Answer from the drawing. Dimensions are ordinates in mm from the lowest x, y and z of the part. Coordinates: 2 decimals unless noted, no trailing zeros. Write each loop counter-clockwise with the first axis right and the second up, starting at its lowest first coordinate (ties: lowest second). Pieces come first, ordered by that corner, then holes. Notation, with made-up numbers: (9.25, 78.25) - (20.25, 78.25) arc R16 ccw to (20.25, 83.25) - close; hole circle Ø1 at (32, -9.75). An arc over 180 degrees is marked (long way). Use CSV: the item, a comma, the result in double quotes. Start each with the question number.
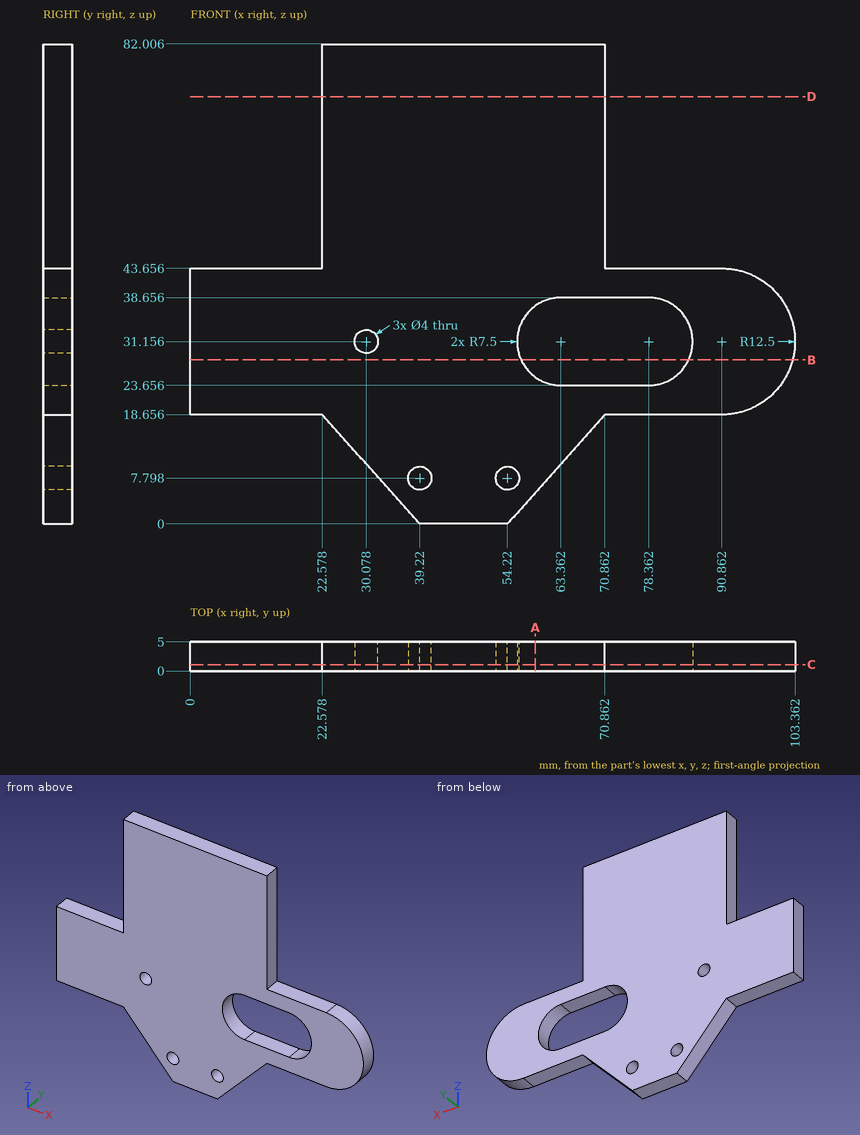
Item 1: A cutting plane is placed at C-C (y = 1.1). Determine the outline of the cut face in (x, z) (1 decimal).
Item 2: A cutting plane is placed at B-B (z = 28). Determine the outline of the cut face in (x, y) (1 decimal).
Item 3: Each of these flat-tipped pins is pushed along its axis until it touches: pin 1 (2.5 mm diameter, centred on x = 78, y = 3, fed in from +Z); pin 2 (1.5 mm diameter, centred on x = 12, y = 3.5, fed in from -Z); pin 3 (2.5 mm diameter, centred on x = 72, y = 1.5, fed in from -Z); pin 4 (2.5 mm diameter, centred on x = 54.22, z = 7.8, fed in from +Y). Where does it stop, or does it pass through?
Item 4: A cutting plane is placed at A-A (x = 59). Determine the outline of the cut face in (y, z) (1 decimal).
Item 5: Straight lines are drawn through the part: probe 1 along Z at (x, y) = (39.5, 0.75) (1 decimal); probe 2 along Z at (x, y) = (72.5, 3.9) (1 decimal); probe 3 along X at (y, z) = (3, 46). For each, find the intervals that lie inside material, in ascending order. Write a range as [from, to].
Item 6: A cutting plane is placed at D-D (z = 73). Determine the outline of the cut face in (x, y).
Calculated:
1,outline,"(0, 18.7) - (22.6, 18.7) - (39.2, 0) - (54.2, 0) - (70.9, 18.7) - (90.9, 18.7) arc R12.5 ccw to (90.9, 43.7) - (70.9, 43.7) - (70.9, 82) - (22.6, 82) - (22.6, 43.7) - (0, 43.7) - close; hole circle Ø4 at (30.1, 31.2); hole circle Ø4 at (39.2, 7.8); hole circle Ø4 at (54.2, 7.8); hole (63.4, 23.7) - (78.4, 23.7) arc R7.5 ccw to (78.4, 38.7) - (63.4, 38.7) arc R7.5 ccw to start"
2,outline,"(0, 0) - (56.6, 0) - (56.6, 5) - (0, 5) - close; (85.2, 0) - (103, 0) - (103, 5) - (85.2, 5) - close"
3,pin 1,"stops at z = 43.66"
3,pin 2,"stops at z = 18.66"
3,pin 3,"stops at z = 18.53"
3,pin 4,"passes through"
4,outline,"(0, 5.4) - (5, 5.4) - (5, 25.1) - (0, 25.1) - close; (0, 37.3) - (5, 37.3) - (5, 82) - (0, 82) - close"
5,probe 1,"z = [0, 5.8], [9.8, 82]"
5,probe 2,"z = [18.7, 23.7], [38.7, 43.7]"
5,probe 3,"x = [22.58, 70.86]"
6,outline,"(22.58, 0) - (70.86, 0) - (70.86, 5) - (22.58, 5) - close"
